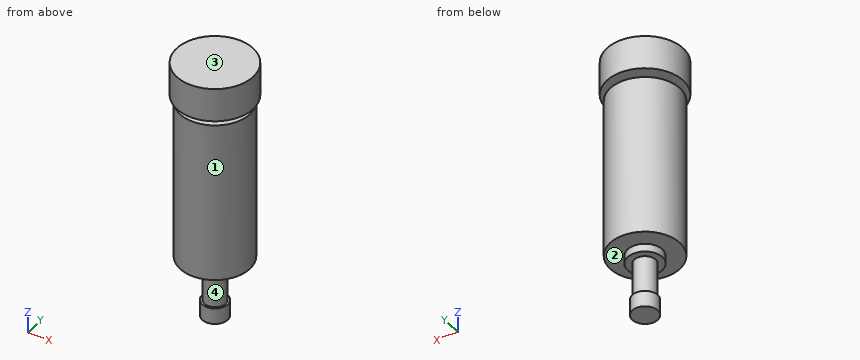
```python
from build123d import *

# Parameters (mm, degrees)
SKETCH_R     = 26
PAD_DEPTH    = 120
SKETCH001_R  = 8
PAD001_DEPTH = 5
SKETCH002_R  = 28.5
PAD002_DEPTH = 25
SKETCH003_R  = 13
PAD003_DEPTH = 6
SKETCH004_R  = 8
PAD004_DEPTH = 28
SKETCH005_R  = 9.5
PAD005_DEPTH = 12


with BuildPart() as part:
    # Sketch → Pad (new body)
    with BuildSketch(Plane.XY):
        Circle(SKETCH_R)
    extrude(amount=PAD_DEPTH)

    # Sketch001 (on Face3 of Pad) → Pad001 (join)
    with BuildSketch(Plane.XY.offset(120)):
        Circle(SKETCH001_R)
    extrude(amount=PAD001_DEPTH)

    # Sketch002 (on Face5 of Pad001) → Pad002 (join)
    with BuildSketch(Plane.XY.offset(125)):
        Circle(SKETCH002_R)
    extrude(amount=PAD002_DEPTH)

    # Sketch003 (on Face7 of Pad002) → Pad003 (join)
    with BuildSketch(Plane(origin=(0, 0, 0), x_dir=(1, 0, 0), z_dir=(0, 0, -1))):
        Circle(SKETCH003_R)
    extrude(amount=PAD003_DEPTH)

    # Sketch004 (on Face9 of Pad003) → Pad004 (join)
    with BuildSketch(Plane(origin=(0, 0, -6), x_dir=(1, 0, 0), z_dir=(0, 0, -1))):
        Circle(SKETCH004_R)
    extrude(amount=PAD004_DEPTH)

    # Sketch005 (on Face11 of Pad004) → Pad005 (join)
    with BuildSketch(Plane(origin=(0, 0, -34), x_dir=(1, 0, 0), z_dir=(0, 0, -1))):
        Circle(SKETCH005_R)
    extrude(amount=PAD005_DEPTH)


solid = part.part
```
Can you work these out from the model? Positions are in its coordinate system, mm. Face numbers are marked on the shaded views. Coordinates: 2 decimals unless noted, no trailing zeros. Loops run counter-clockwise (first coordinate to the right, second up) from the corner with the lowest first, then second, coordinate; pieces in that order, holes last. Notation, with made-up numbers: (25.5, -33.5) -> (63.5, -33.5) arc R38 cw to (63.5, 4.5) -> close; hole circle Ø3 at (-10, -9.75). An arc over 180 degrees is marked (long way). Answer as a JSON object with one key per item and string values.
1) If I drill on line 1 (Z direction, x = -3, y = 10.5); line 2 (Z direction, x = 15.5, y = -7); line 3 (X direction, y = -1, z = 57.5), over which ranges is the centre line in solid material (lowest first)?
Results:
{"line 1": "z = -6 to 120, 125 to 150", "line 2": "z = 0 to 120, 125 to 150", "line 3": "x = -25.98 to 25.98"}
2) Imagine slicing it at C-C (y = -16.5). Please give me the cut outline in (x, z), then the cut area to 3 significant figures.
Results:
{"outline": "(-23.24, 125) -> (23.24, 125) -> (23.24, 150) -> (-23.24, 150) -> close; (-20.09, 0) -> (20.09, 0) -> (20.09, 120) -> (-20.09, 120) -> close", "area": "5,980 mm^2"}
3) Imagine slicing it at B-B (x = 22). Please give me the cut outline in (y, z), then the cut area to 3 significant figures.
Results:
{"outline": "(-18.12, 125) -> (18.12, 125) -> (18.12, 150) -> (-18.12, 150) -> close; (-13.86, 0) -> (13.86, 0) -> (13.86, 120) -> (-13.86, 120) -> close", "area": "4,230 mm^2"}
4) For P1, Ø8, axis at x = -2.5, y = -14, coming from the -Z side; P2, Ø4, axis at y = -19.5, z = 109, coming from the +X side; P3, Ø6, axis at y = 1, z = -8, coming from the +X side, each with a flat end and sliding along its axis, tell me the tip position at first contact or that it passes through.
Results:
{"P1": "stops at z = -6", "P2": "stops at x = 19.23", "P3": "stops at x = 13"}
5) Thinking about a two-plate mould opening in Z: for the marked faces 1, 2, 3 and 4, which applies, pulls with the +Z half, pulls with the -Z half, needs draft (parallel to the pull), parting line crosses it, or undercut?
Results:
{"face 1": "needs draft", "face 2": "pulls with the -Z half", "face 3": "pulls with the +Z half", "face 4": "undercut"}
6) Imagine slicing it at A-A (y = 0). Please give me the cut outline in (x, z).
Results:
{"outline": "(-28.5, 125) -> (-8, 125) -> (-8, 120) -> (-26, 120) -> (-26, 0) -> (-13, 0) -> (-13, -6) -> (-8, -6) -> (-8, -34) -> (-9.5, -34) -> (-9.5, -46) -> (9.5, -46) -> (9.5, -34) -> (8, -34) -> (8, -6) -> (13, -6) -> (13, 0) -> (26, 0) -> (26, 120) -> (8, 120) -> (8, 125) -> (28.5, 125) -> (28.5, 150) -> (-28.5, 150) -> close"}
7) Imagine slicing it at D-D (z = -4). Please give me the cut outline in (x, y), then the cut area to 3 significant figures.
Results:
{"outline": "circle Ø26 at (0, 0)", "area": "531 mm^2"}
